from build123d import *

# Parameters (mm, degrees)
F0_W     = 37.869452
F0_H     = 6.726544
F1_DEPTH = 19.05


with BuildPart() as f1:
    # F0 (on Front) → F1 (new body)
    with BuildSketch(Plane.XZ):
        Polygon((-59.760556, 47.031272), (-70.955373, 47.031272), (-70.955373, -55.858262), (-59.760556, -55.858262), (-59.760556, -49.902789), (-59.760556, 40.296745), (-59.760556, 47.023289), align=None)
        Polygon((-9.379123, 47.023289), (-21.891104, 47.023289), (-21.891104, 40.296745), (-21.891104, -49.902789), (-21.891104, -55.730475), (-9.379123, -55.730475), align=None)
        Polygon((-59.760556, -49.902789), (-59.760556, -55.858262), (-21.891104, -55.858262), (-21.891104, -55.730475), (-21.891104, -49.902789), align=None)
        with Locations((-40.82583, 43.660017)):
            Rectangle(F0_W, F0_H)
    extrude(amount=F1_DEPTH)


solid = f1.part
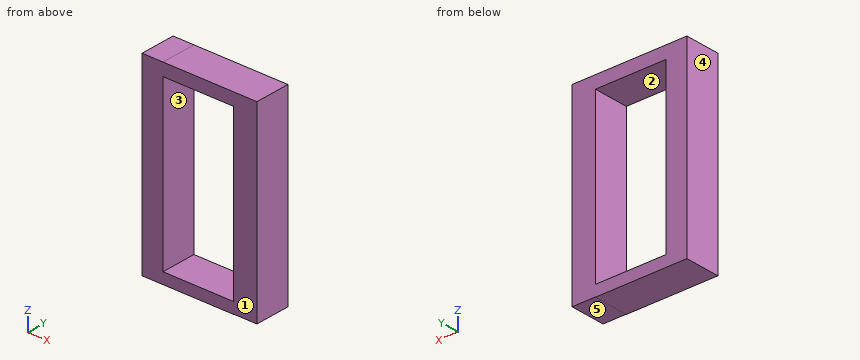
Verification items for the finished model (mm, model axes). Face numbers are marked on the shaded views. A direction names the side the tool comes from. Give positions to 0.01 mm unless a question says otherwise; leave off trailing zeros. Write each loop counter-clockwise with the first axis right and the second up, starting at its lowest first coordinate (ties: lowest second). Pieces come first, ordered by that corner, then holes. Notation, with made-up numbers: M -2.75,-22.5 L 35.25,-22.5 A9 cw 35.25,-12.5 Z; hole C 22,-27.75 d11. An arc over 180 degrees is marked long. Put each result on its own line as item: value. Start each with the question number.
1. Draft check along X on the marked faces 3, 4 and 5. Enter one of: +X half, -X half, draft (parallel to the pull), parting line (faces both ways), or undercut.
2. Go/stop test with flat-tipped pins: pin 1 Ø5.5 at (x, y) = (-32, -12) entering from +Z; pin 2 Ø4 at (x, z) = (-24, 22) entering from +Y. Record where each tip stops, or that it passes through.
3. Section check C-C (z = -40). Record the cut outline in (x, y).
4. Scan lines: line 1 along Z through (x, y) = (-59.5, -14.75); line 2 along X through (y, z) = (-16.75, 31); line 3 along Z through (x, y) = (-19, -17). Record each from-to range of solid material in increasing order. Write a range as [from, to].
5. Section check B-B (x = -25). Record the cut outline in (y, z), and give its area (3 significant figures).
6. Set-up check for the marked faces 1 and 2: record each of +Z, -Z, +X, -X, +Y, -Y from which the full face is reachable in a straight line by a thin tool's end or side.
Answer list:
1. face 3: undercut
1. face 4: -X half
1. face 5: draft
2. pin 1: z = 47.02
2. pin 2: through
3. outline: M -70.96,-19.05 L -59.76,-19.05 L -59.76,0 L -70.96,0 Z; M -21.89,-19.05 L -9.38,-19.05 L -9.38,0 L -21.89,0 Z
4. line 1: [-55.86, -49.9], [40.3, 47.02]
4. line 2: [-70.96, -59.76], [-21.89, -9.38]
4. line 3: [-55.73, 47.02]
5. outline: M -19.05,-55.86 L 0,-55.86 L 0,-49.9 L -19.05,-49.9 Z; M -19.05,40.3 L 0,40.3 L 0,47.02 L -19.05,47.02 Z
5. area: 242 mm2
6. face 1: +Z, -Z, +X, -X, -Y
6. face 2: +Y, -Y
